```python
from build123d import *

# Parameters (mm, degrees)
F1_DEPTH = 50
F2_W     = 240
F2_H     = 110
F2_R     = 50
F3_DEPTH = 35
F5_DEPTH = 80


with BuildPart() as f1:
    # F0 (on Top) → F1 (new body)
    with BuildSketch(Plane.XY):
        Polygon((120, 70), (0, 70), (-120, 70), (-120, -70), (120, -70), align=None)
        with BuildLine():
            ThreePointArc((0, 50), (35.3553390593, 35.3553390593), (50, 0))
            ThreePointArc((50, 0), (-35.3553390593, -35.3553390593), (0, 50))
        make_face(mode=Mode.SUBTRACT)
    extrude(amount=-F1_DEPTH)

    # F2 (on face) → F3 (join)
    with BuildSketch(Plane(origin=(0, 0, -50), x_dir=(1, 0, 0), z_dir=(0, 0, -1))):
        Rectangle(F2_W, F2_H)
        Circle(F2_R, mode=Mode.SUBTRACT)
        Circle(F2_R)
    extrude(amount=F3_DEPTH)

    # F4 (on Front) → F5 (join, symmetric)
    with BuildSketch(Plane.XZ):
        Polygon((161.9289219379, -39.3364913762), (120.1279684901, -23.6113723367), (119.9289113283, -84.9194303155), (161.9289219379, -71.184836328), align=None)
    extrude(amount=F5_DEPTH, both=True)


solid = f1.part
```
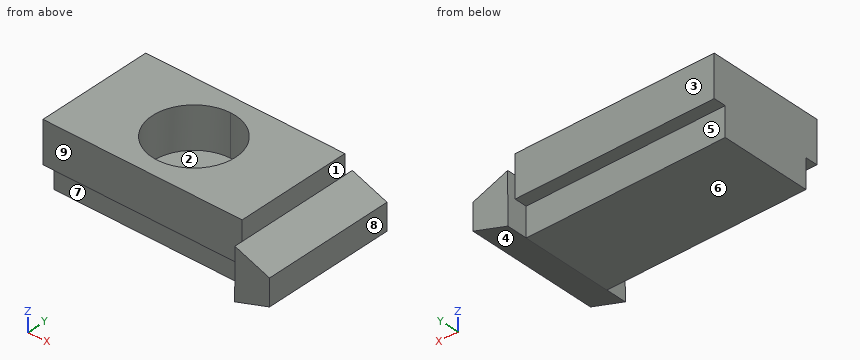
The listing builds one solid part. Answer for the finished solid, in the listing's coordinates (mm). Face numbers are marked on the shaded views. A direction names the side the tool comes from. Round coordinates to 2 decimals unless told otherwise and drop trailing zeros. Loops run counter-clockwise (first coordinate to the right, second up) from the corner with the lowest first, then second, coordinate; pieces in that order, holes last. Notation, with made-up numbers: (55, -33) - (67, -33) arc R21 cw to (67, -29) - close; hole circle Ø3 at (88, -11.5). An arc over 180 degrees is marked (long way). Use one line per item in the form item = value. Start each with the question number.
1. The part is cut by section D-D on y = 23.5. Determine the outline of the cut face in (x, z).
2. A tool of negligible diameter and unlimited length cuts with its end or side. For the marked faces 5, 6, 7, 8 and 9, from which of +Z, -Z, +X, -X, +Y, -Y can it reach the whole face along a straight path? Write none if from no direction.
3. The part is cut by section A-A on x = 71.5. Determine the outline of the cut face in (y, z), then the cut area to 4 significant figures.
4. For a pull along X with two mould halves and no side action, classify the marked faces 1, 2, 3 and 4 as pulls with the +X half, pulls with the -X half, needs draft (parallel to the pull), parting line crosses it, or undercut.
5. The part is cut by section B-B on z = -58.5. Determine the outline of the cut face in (x, y), then the cut area to 3 significant figures.
6. Consider line 1 (X direction, y = 0, z = -21); line 2 (Z direction, x = -12, y = 10); line 3 (Y direction, x = -106.5, z = -59.5). Determine where each line is inside the solid, lowest interval first. Write a range as [from, to].
7. The part is cut by section C-C on y = -39.5. Determine the outline of the cut face in (x, z).
8. Given pin 1 Ø25 at (x, z) = (-52.5, -16) entering from +Y; pin 2 Ø1 at (y, z) = (-56, -56) entering from -X; pin 3 Ø1 at (x, y) = (85.5, 27.5) entering from +Z; pin 4 Ø10 at (x, z) = (43.5, -67) entering from -Y, each flat-ended and moving along its own axis, determine where each tip first touches the part or whether it passes through.
Geometry check:
q1.outline = (-120, -85) - (120, -85) - (120, -84.9) - (161.93, -71.18) - (161.93, -39.34) - (120.13, -23.61) - (120, -63.02) - (120, 0) - (44.13, 0) - (44.13, -50) - (-44.13, -50) - (-44.13, 0) - (-120, 0) - close
q2.face_5 = -Z, -X, +Y
q2.face_6 = -Z, +X, -X, +Y, -Y
q2.face_7 = -Z, -X, -Y
q2.face_8 = +Z, -Z, +X, +Y, -Y
q2.face_9 = +Z, -Z, -X, -Y
q3.outline = (-70, -50) - (-55, -50) - (-55, -85) - (55, -85) - (55, -50) - (70, -50) - (70, 0) - (-70, 0) - close
q3.area = 10,850 mm^2
q4.face_1 = undercut
q4.face_2 = undercut
q4.face_3 = needs draft
q4.face_4 = pulls with the +X half
q5.outline = (-120, -55) - (120, -55) - (120, 55) - (-120, 55) - close; (120.01, -80) - (161.93, -80) - (161.93, 80) - (120.01, 80) - close
q5.area = 33,100 mm^2
q6.line_1 = [-120, -50], [50, 120]
q6.line_2 = [-85, -50]
q6.line_3 = [-55, 55]
q7.outline = (-120, -85) - (120, -85) - (120, -84.9) - (161.93, -71.18) - (161.93, -39.34) - (120.13, -23.61) - (120, -63.02) - (120, 0) - (30.66, 0) - (30.66, -50) - (-30.66, -50) - (-30.66, 0) - (-120, 0) - close
q8.pin_1 = 70
q8.pin_2 = 120.02
q8.pin_3 = 0
q8.pin_4 = -55
